Read the model definition and answer for the solid it produces. Units are mm, in the model's axes. A direction names the side the tool comes from. Coordinates: 2 decimals unless noted, no trailing zeros. Write each loop counter-clockwise with the first axis right and the second up, starting at its lowest first coordinate (ties: lowest second). Pieces come first, ordered by that corner, then holes. Notation, with made-up numbers: (45.5, -12.75) -> (89.5, -12.75) arc R16 cw to (89.5, -3.75) -> close; hole circle Ø8 at (-6, 27.5). An arc over 180 degrees is marked (long way). Answer as a JSON object with one key per item and string values. Group by question number.
(1) Find section B-B (x = 17). Give the vertices of the cut face in (y, z).
(2) Flat-ended cylindrical pins translate along their axes: P1, Ø4, axis at x = 9.5, z = 21, coming from the +Y side; P2, Ø1, axis at x = 19.5, y = 13, coming from the +Z side; P3, Ø12, axis at y = 17, z = 11, coming from the +X side; P4, Ø3, axis at y = 9.5, z = 3, coming from the -X side. Find the tip coordinate at first contact, or state that the pin passes through.
(3) Straight lines are drawn through the part: L1, parallel to X at y = 21, z = 23; L2, parallel to X at y = 55.5, z = 7.75; L3, parallel to Y at x = 32.5, z = 24.5. For each, find the intervals that lie inside material, in ascending order.
(4) Find section C-C (z = 3.25). Give the vertices of the cut face in (x, y), then the cut area to 3 significant figures.
(5) Find section A-A (z = 18.75). Give the vertices of the cut face in (x, y).
(6) Which of the six approach directions +Z, -Z, +X, -X, +Y, -Y give full straight-line access (tool end or side, diameter ignored) to faces 1 (the face through (34, 24, 9)), 2 (the face through (17, 35, 16)), 3 (the face through (7, 17, 24)), 4 (the face through (11, 63, 5))?
(7) For a pull along X with two mould halves and no side action, classify faces 5 (the face through (23, 63, 5)), 6 (the face through (-3, 17, 24)), 7 (the face through (39, 17, 27)) as +X half, -X half, draft (parallel to the pull), parting line (faces both ways), or undercut.
(8) Find section D-D (y = 49). Give the vertices of the cut face in (x, z), then the cut area to 3 significant figures.
Autodesk Inventor part; units mm, degrees
ref_plane "YZ Plane" through (0, 0, 0) normal (1, 0, 0) x (0, 1, 0)
ref_plane "XZ Plane" through (0, 0, 0) normal (0, 1, 0) x (-1, 0, 0)
ref_plane "XY Plane" through (0, 0, 0) normal (0, 0, 1) x (1, 0, 0)
sketch "Náčrt1" plane through (0, 0, 0) normal (0, 0, 1) x (1, 0, 0)
  line L0 (0, 0) -> (0, 60)
  line L1 (5, 75) -> (0, 60)
  line L2 (5, 75) -> (11, 75)
  line L3 (11, 75) -> (11, 51)
  arc A0 (11, 51) -> (23, 51) centre (17, 51) ccw
  line L4 (23, 51) -> (23, 75)
  line L5 (23, 75) -> (29, 75)
  line L6 (34, 60) -> (29, 75)
  line L7 (34, 60) -> (34, 0)
  line L8 (34, 0) -> (0, 0)
  dimension "d0" = 60
  dimension "d3" = 6
  dimension "d4" = 24
  dimension "d5" = 12
  dimension "d6" = 6
extrude "Vysunutí1" add sketch "Náčrt1" along normal blind 10
sketch "Náčrt2" plane through (0, 0, 0) normal (0, -1, 0) x (1, 0, 0)
  line L0 (5, 10) -> (0, 10)
  line L1 (34, 0) -> (34, 10)
  line L2 (0, 10) -> (34, 10)
  line L3 (34, 10) -> (34, 24)
  line L4 (34, 24) -> (39, 24)
  line L5 (39, 24) -> (39, 30)
  line L6 (-5, 30) -> (-5, 24)
  line L7 (-5, 24) -> (0, 24)
  line L8 (0, 24) -> (0, 10)
  line L9 (-5, 30) -> (7, 30)
  line L10 (7, 30) -> (7, 18)
  line L11 (7, 18) -> (27, 18)
  line L12 (27, 18) -> (27, 30)
  line L13 (27, 30) -> (39, 30)
  point P0 (0, 0)
  dimension "d11" = 14
  dimension "d12" = 5
  dimension "d13" = 6
  dimension "d14" = 44
  dimension "d15" = 6
  dimension "d16" = 12
  dimension "d17" = 12
  dimension "d18" = 20
extrude "Vysunutí2" add sketch "Náčrt2" against normal blind 35
properties part number "6"
Results below:
{
 "1": {"outline": "(0, 0) -> (45, 0) -> (45, 10) -> (35, 10) -> (35, 18) -> (0, 18) -> close"},
 "2": {"P1": "passes through", "P2": "stops at z = 18", "P3": "stops at x = 34", "P4": "stops at x = 0"},
 "3": {"L1": "x = 0 to 7, 27 to 34", "L2": "x = 0 to 11, 23 to 34", "L3": "y = 0 to 35"},
 "4": {"outline": "(0, 0) -> (34, 0) -> (34, 60) -> (29, 75) -> (23, 75) -> (23, 51) arc R6 cw to (11, 51) -> (11, 75) -> (5, 75) -> (0, 60) -> close", "area": "2,130 mm2"},
 "5": {"outline": "(0, 0) -> (7, 0) -> (7, 35) -> (0, 35) -> close; (27, 0) -> (34, 0) -> (34, 35) -> (27, 35) -> close"},
 "6": {"face 1": "-Z, +X, +Y, -Y", "face 2": "+Z, +X, -X, +Y", "face 3": "+Z, +Y, -Y", "face 4": "+Z, -Z, +Y"},
 "7": {"face 5": "undercut", "face 6": "draft", "face 7": "+X half"},
 "8": {"outline": "(0, 0) -> (11.34, 0) -> (11.34, 10) -> (0, 10) -> close; (22.66, 0) -> (34, 0) -> (34, 10) -> (22.66, 10) -> close", "area": "227 mm2"}
}
